from build123d import *

# Parameters (mm, degrees)
SKETCH1_R               = 3
BOSS_EXTRUDE1_DEPTH     = 5
SKETCH1_3_R             = 3
BOSS_EXTRUDE2_DEPTH     = 7.5
SKETCH1_4_R             = 2.5
BOSS_EXTRUDE3_DEPTH     = 12.5
BOSS_EXTRUDE4_DEPTH     = 8
CUT_EXTRUDE1_DEPTH      = 23.989127865
CUT_EXTRUDE1_DEPTH_BACK = 23.989127865
SKETCH6_W               = 10
SKETCH6_H               = 10
SKETCH7_R               = 3
CUT_EXTRUDE2_DEPTH      = 27.786190472
FILLET4_R               = 2.5
FILLET5_R               = 3
FILLET6_R               = 2


# Some blends are built 0.0001 mm under size
with BuildPart() as part:
    # Sketch1 → Boss-Extrude1 (new, symmetric)
    with BuildSketch(Plane.XY):
        with BuildLine():
            ThreePointArc((0, 5), (5, 0), (0, -5))
            Line((0, -5), (-5, -5))
            Line((-5, -5), (-5, 5))
            Line((-5, 5), (0, 5))
        make_face()
        Circle(SKETCH1_R, mode=Mode.SUBTRACT)
    extrude(amount=BOSS_EXTRUDE1_DEPTH, both=True)

    # Sketch1<3> → Boss-Extrude2 (add, symmetric)
    with BuildSketch(Plane.XY):
        Circle(SKETCH1_3_R)
    extrude(amount=BOSS_EXTRUDE2_DEPTH, both=True)

    # Sketch1<4> → Boss-Extrude3 (add, symmetric)
    with BuildSketch(Plane.XY):
        Circle(SKETCH1_4_R)
    extrude(amount=BOSS_EXTRUDE3_DEPTH, both=True)

    # Sketch5 → Boss-Extrude4 (add, symmetric)
    with BuildSketch(Plane.XY):
        with BuildLine():
            Line((-5, 5), (-5, -5))
            Line((-5, -5), (-11.5, -5))
            ThreePointArc((-11.5, -5), (-16.5, 0), (-11.5, 5))
            Line((-11.5, 5), (-5, 5))
        make_face()
    extrude(amount=BOSS_EXTRUDE4_DEPTH, both=True)

    # Sketch6 → Cut-Extrude1 (cut, two sides: drawn at the far end of the back side and taken through both)
    with BuildSketch(Plane(origin=(0, 5, 0), x_dir=(1, 0, 0), z_dir=(0, 1, 0)).offset(-CUT_EXTRUDE1_DEPTH_BACK)):
        with Locations((-11.5, 0)):
            Rectangle(SKETCH6_W, SKETCH6_H)
    extrude(amount=CUT_EXTRUDE1_DEPTH + CUT_EXTRUDE1_DEPTH_BACK, mode=Mode.SUBTRACT)

    # Sketch7 → Cut-Extrude2 (cut, through all)
    with BuildSketch(Plane(origin=(0, 0, -8), x_dir=(-1, 0, 0), z_dir=(0, 0, -1))):
        with Locations((11.5, 0)):
            Circle(SKETCH7_R)
    extrude(amount=-CUT_EXTRUDE2_DEPTH, mode=Mode.SUBTRACT)

    # Fillet4
    # the kernel refuses this fillet: 2.5 mm, written as the material it adds along each edge
    with BuildSketch(Plane(origin=(-5, -5, 5), x_dir=(0, 0, 1), z_dir=(0, 1, 0)), Plane(origin=(-5, -5, -5), x_dir=(1, 0, 0), z_dir=(0, 1, 0))) as fillet4_piece_1:
        with BuildLine():
            CenterArc((FILLET4_R, FILLET4_R), FILLET4_R, 180, 90)
            Line((0, FILLET4_R), (0, 0))
            Line((0, 0), (FILLET4_R, 0))
        make_face()
    extrude(amount=10)

    # Fillet5
    fillet5_edges = [part.edges().sort_by_distance(p)[0] for p in [
        (-5, 0, -8),
        (-5, 0, 8),
    ]]
    fillet(fillet5_edges, radius=FILLET5_R)

    # Fillet6
    fillet6_edges = [part.edges().sort_by_distance(p)[0] for p in [
        (-6.5, 0, -5),
        (-6.5, 0, 5),
    ]]
    fillet(fillet6_edges, radius=FILLET6_R - 0.0001)  # a hair under: the kernel refuses the full size


solid = part.part
Geometry check sheet. Reference: the model listing, model coordinates, mm. A direction names the side the tool comes from. Round coordinates to 2 decimals unless told otherwise and drop trailing zeros. Loops run counter-clockwise (first coordinate to the right, second up) from the corner with the lowest first, then second, coordinate; pieces in that order, holes last.
Item 1: Cross-section at C-C on z = 4.5. Record the boundary of the cut face in (x, y).
Item 2: Access from +Z, -Z, +X, -X, +Y, -Y to the whole of each face (thin tool, end or side, straight path). Record for faces 5 (the flat face through (-6, -5, 0)), 6 (the flat face through (-2, 2, -7.5)), 7 (the cylindrical face through (-0.54, -2.44, 10.04)).
Item 3: Cross-section at B-B on y = 1. Count the separate pieces of the cut face and the enclosed holes in it, then the cut area to 3 significant figures.
Item 4: Cross-section at A-A on x = -12.75. Record the boundary of the cut face in (y, z), then the cut area to 3 significant figures.
Item 5: Thickness scan on line 1 (Z direction, x = -15.25, y = 1); line 2 (Y direction, x = -11.5, z = 5.85); line 3 (Z direction, x = -7.5, y = -4). Record the ranges inside material, lowest first.
Item 6: Mould release check, pull along Z, two halves, no side actions. Record for faces 1 (the flat face through (-14, -2, 8)), 2 (the flat face through (-6.5, 0, 0)), 3 (the flat face through (-14, -2, -8)), 4 (the cylindrical face through (-7.1, 0.07, 4.43)): pulls with the +Z half, pulls with the -Z half, needs draft (parallel to the pull), parting line crosses it, or undercut.
Item 7: Gauge pin test, flat ends, axial feed: pin 1 (2 mm diameter, centred on y = -1.5, z = -3.5, fed in from -X); pin 2 (2.5 mm diameter, centred on x = -14.5, y = -2, fed in from -Z); pin 3 (3 mm diameter, centred on y = 0.5, z = -0.5, fed in from -X). Record the tip position at first contact, or that the pin passes through.
Answer sheet:
1. outline: (-7.18, -5) - (0, -5) arc R5 ccw to (0, 5) - (-7.18, 5) - close
2. face 5: +Z, -Z, +X, -X, -Y
2. face 6: -Z
2. face 7: +Z
3. separate pieces: 3
3. enclosed holes: 0
3. area: 225 mm2
4. outline: (-4.84, -8) - (-2.73, -8) - (-2.73, -5) - (-4.84, -5) - close; (-4.84, 5) - (-2.73, 5) - (-2.73, 8) - (-4.84, 8) - close; (2.73, -8) - (4.84, -8) - (4.84, -5) - (2.73, -5) - close; (2.73, 5) - (4.84, 5) - (4.84, 8) - (2.73, 8) - close
4. area: 25.4 mm2
5. line 1: z = -8 to -5, 5 to 8
5. line 2: y = -5 to -3, 3 to 5
5. line 3: z = -8 to -4.73, 4.73 to 8
6. face 1: pulls with the +Z half
6. face 2: undercut
6. face 3: pulls with the -Z half
6. face 4: undercut
7. pin 1: stops at x = -7.18
7. pin 2: stops at z = -8
7. pin 3: stops at x = -6.5
